from build123d import *

# Parameters (mm, degrees)
SKETCH1_W           = 11.5
SKETCH1_H           = 7.8
BOSS_EXTRUDE1_DEPTH = 300
SKETCH2_W           = 0.835250229
SKETCH2_H           = 1.6
CUT_EXTRUDE1_DEPTH  = 301.080443381
SKETCH3_R           = 3
CUT_EXTRUDE2_DEPTH  = 4.7
SKETCH4_R           = 1.7
CUT_EXTRUDE3_DEPTH  = 301.091906755


with BuildPart() as part:
    # Sketch1 → Boss-Extrude1 (new body)
    with BuildSketch(Plane.XY):
        Rectangle(SKETCH1_W, SKETCH1_H)
    extrude(amount=BOSS_EXTRUDE1_DEPTH)

    # Sketch2 → Cut-Extrude1 (cut, through all)
    with BuildSketch(Plane.XY.offset(300)):
        with Locations((5.332374886, 1.7)):
            Rectangle(SKETCH2_W, SKETCH2_H)
        with Locations((-5.332374886, 1.7)):
            Rectangle(SKETCH2_W, SKETCH2_H)
    extrude(amount=-CUT_EXTRUDE1_DEPTH, mode=Mode.SUBTRACT)

    # Sketch3 → Cut-Extrude2 (cut)
    with BuildSketch(Plane(origin=(0, 3.9, 0), x_dir=(1, 0, 0), z_dir=(0, 1, 0))):
        with Locations(Location((0, -288.4, 0), (0, 0, 270))):
            Circle(SKETCH3_R)
        with Locations(Location((0, -263.4, 0), (0, 0, 270))):
            Circle(SKETCH3_R)
        with Locations(Location((0, -238.4, 0), (0, 0, 270))):
            Circle(SKETCH3_R)
        with Locations(Location((0, -213.4, 0), (0, 0, 270))):
            Circle(SKETCH3_R)
        with Locations(Location((0, -188.4, 0), (0, 0, 270))):
            Circle(SKETCH3_R)
        with Locations(Location((0, -163.4, 0), (0, 0, 270))):
            Circle(SKETCH3_R)
        with Locations(Location((0, -138.4, 0), (0, 0, 270))):
            Circle(SKETCH3_R)
        with Locations(Location((0, -113.4, 0), (0, 0, 270))):
            Circle(SKETCH3_R)
        with Locations(Location((0, -88.4, 0), (0, 0, 270))):
            Circle(SKETCH3_R)
        with Locations(Location((0, -63.4, 0), (0, 0, 270))):
            Circle(SKETCH3_R)
        with Locations(Location((0, -38.4, 0), (0, 0, 270))):
            Circle(SKETCH3_R)
        with Locations(Location((0, -13.4, 0), (0, 0, 270))):
            Circle(SKETCH3_R)
        with Locations((0, 11.6)):
            Circle(SKETCH3_R)
        with Locations((0, 36.6)):
            Circle(SKETCH3_R)
        with Locations((0, 61.6)):
            Circle(SKETCH3_R)
        with Locations((0, 86.6)):
            Circle(SKETCH3_R)
        with Locations((0, 111.6)):
            Circle(SKETCH3_R)
        with Locations((0, 136.6)):
            Circle(SKETCH3_R)
        with Locations((0, 161.6)):
            Circle(SKETCH3_R)
        with Locations((0, 186.6)):
            Circle(SKETCH3_R)
        with Locations((0, 211.6)):
            Circle(SKETCH3_R)
        with Locations((0, 236.6)):
            Circle(SKETCH3_R)
        with Locations((0, 261.6)):
            Circle(SKETCH3_R)
        with Locations((0, 286.6)):
            Circle(SKETCH3_R)
        with Locations((0, 311.6)):
            Circle(SKETCH3_R)
        with Locations((0, 336.6)):
            Circle(SKETCH3_R)
        with Locations((0, 361.6)):
            Circle(SKETCH3_R)
        with Locations((0, 386.6)):
            Circle(SKETCH3_R)
        with Locations((0, 411.6)):
            Circle(SKETCH3_R)
        with Locations((0, 436.6)):
            Circle(SKETCH3_R)
    extrude(amount=-CUT_EXTRUDE2_DEPTH, mode=Mode.SUBTRACT)

    # Sketch4 → Cut-Extrude3 (cut, through all)
    with BuildSketch(Plane(origin=(0, -0.8, 0), x_dir=(1, 0, 0), z_dir=(0, 1, 0))):
        with Locations(Location((0, -288.4, 0), (0, 0, 270))):
            Circle(SKETCH4_R)
        with Locations(Location((0, -263.4, 0), (0, 0, 270))):
            Circle(SKETCH4_R)
        with Locations(Location((0, -238.4, 0), (0, 0, 270))):
            Circle(SKETCH4_R)
        with Locations(Location((0, -213.4, 0), (0, 0, 270))):
            Circle(SKETCH4_R)
        with Locations(Location((0, -188.4, 0), (0, 0, 270))):
            Circle(SKETCH4_R)
        with Locations(Location((0, -163.4, 0), (0, 0, 270))):
            Circle(SKETCH4_R)
        with Locations(Location((0, -138.4, 0), (0, 0, 270))):
            Circle(SKETCH4_R)
        with Locations(Location((0, -113.4, 0), (0, 0, 270))):
            Circle(SKETCH4_R)
        with Locations(Location((0, -88.4, 0), (0, 0, 270))):
            Circle(SKETCH4_R)
        with Locations(Location((0, -63.4, 0), (0, 0, 270))):
            Circle(SKETCH4_R)
        with Locations(Location((0, -38.4, 0), (0, 0, 270))):
            Circle(SKETCH4_R)
        with Locations(Location((0, -13.4, 0), (0, 0, 270))):
            Circle(SKETCH4_R)
        with Locations((0, 11.6)):
            Circle(SKETCH4_R)
        with Locations((0, 36.6)):
            Circle(SKETCH4_R)
        with Locations((0, 61.6)):
            Circle(SKETCH4_R)
        with Locations((0, 86.6)):
            Circle(SKETCH4_R)
        with Locations((0, 111.6)):
            Circle(SKETCH4_R)
        with Locations((0, 136.6)):
            Circle(SKETCH4_R)
        with Locations((0, 161.6)):
            Circle(SKETCH4_R)
        with Locations((0, 186.6)):
            Circle(SKETCH4_R)
        with Locations((0, 211.6)):
            Circle(SKETCH4_R)
        with Locations((0, 236.6)):
            Circle(SKETCH4_R)
        with Locations((0, 261.6)):
            Circle(SKETCH4_R)
        with Locations((0, 286.6)):
            Circle(SKETCH4_R)
        with Locations((0, 311.6)):
            Circle(SKETCH4_R)
        with Locations((0, 336.6)):
            Circle(SKETCH4_R)
        with Locations((0, 361.6)):
            Circle(SKETCH4_R)
        with Locations((0, 386.6)):
            Circle(SKETCH4_R)
        with Locations((0, 411.6)):
            Circle(SKETCH4_R)
        with Locations((0, 436.6)):
            Circle(SKETCH4_R)
    extrude(amount=-CUT_EXTRUDE3_DEPTH, mode=Mode.SUBTRACT)


solid = part.part
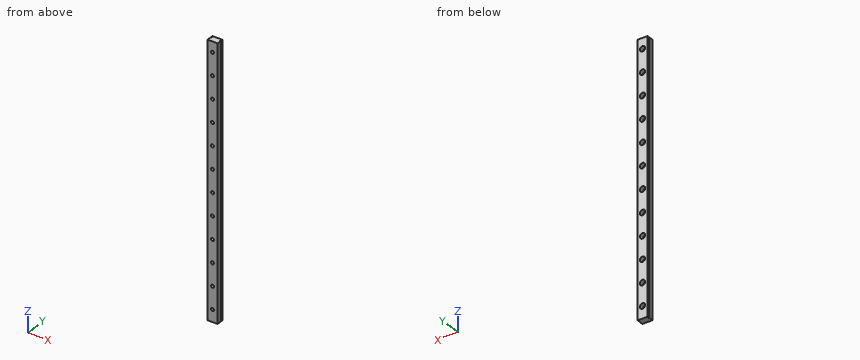
Part model, mm, in its own coordinate system. Give positions to 0.01 mm unless a question says otherwise; leave off trailing zeros. Write each loop counter-clockwise with the first axis right and the second up, starting at its lowest first coordinate (ties: lowest second). Pieces come first, ordered by that corner, then holes.
1) Probe L1, parallel to X at y = 1, z = 139; L2, parallel to X at y = -1.8, z = 38.4; L3, parallel to Y at x = 1.75, z = 62. List the from-to ranges inside material, lowest first.
Resolved:
L1: x = -4.91 to -2.94, 2.94 to 4.91
L2: x = -5.75 to -1.7, 1.7 to 5.75
L3: y = -3.9 to -0.8
2) Cut at A-A on z = 250.5. Write the cut outline in (x, y), then the cut area to 3 significant figures.
Resolved:
outline: (-5.75, -3.9) - (5.75, -3.9) - (5.75, 0.9) - (4.91, 0.9) - (4.91, 2.5) - (5.75, 2.5) - (5.75, 3.9) - (-5.75, 3.9) - (-5.75, 2.5) - (-4.91, 2.5) - (-4.91, 0.9) - (-5.75, 0.9) - close
area: 87.0 mm2
3) Pin check, flat tips, straight feed: pin 1 (6.5 mm diameter, centred on x = -1.5, z = 263, fed in from +Y); pin 2 (4 mm diameter, centred on x = 0, z = 213.4, fed in from +Y). Stop position of each tip, or through.
Resolved:
pin 1: stops at y = 3.9
pin 2: stops at y = -0.8
